Study the drawing (mm; zero at the part's minimum x, y, z) and answer. Round coordinates to 2 decimals unless told otherwise and drop trailing zeros. Loops run counter-clockwise (first coordinate to the right, second up) from the corner with the lowest first, then second, coordinate; pieces in that order, holes last. Notation, with made-up numbers: (70.5, -29) -> (115.5, -29) arc R30 ccw to (115.5, -2) -> close; hole circle Ø9 at (69, 9). An arc over 180 degrees is marked (long way). Write each question's results on one line, items separated by ' | '. Start each with the question number.
(1) The part is cut by section A-A (y = 2.5). Count the separate pieces of the cut face and the enclosed holes in it, plus the area to 3 significant figures.
(2) The part is cut by section C-C (z = 41). Determine the outline of the cut face in (x, y), plus the area to 3 significant figures.
(3) Straight lines are drawn through the part: probe 1 along Z at (x, y) = (123, 6.25); probe 2 along Z at (x, y) = (98, 2.25). For each, find the intervals that lie inside material, in ascending order.
(4) Flat-ended cylindrical pins translate along their axes: pin 1 (1.5 mm diameter, centred on y = 2.5, z = 28, fed in from +X); pin 2 (3 mm diameter, centred on y = 0.5, z = 47, fed in from +X); pin 3 (3 mm diameter, centred on y = 5.5, z = 72, fed in from +X). Find the tip coordinate at first contact, or state that the pin passes through.
(5) The part is cut by section B-B (x = 156.5). Determine the outline of the cut face in (y, z), plus the area to 3 significant figures.
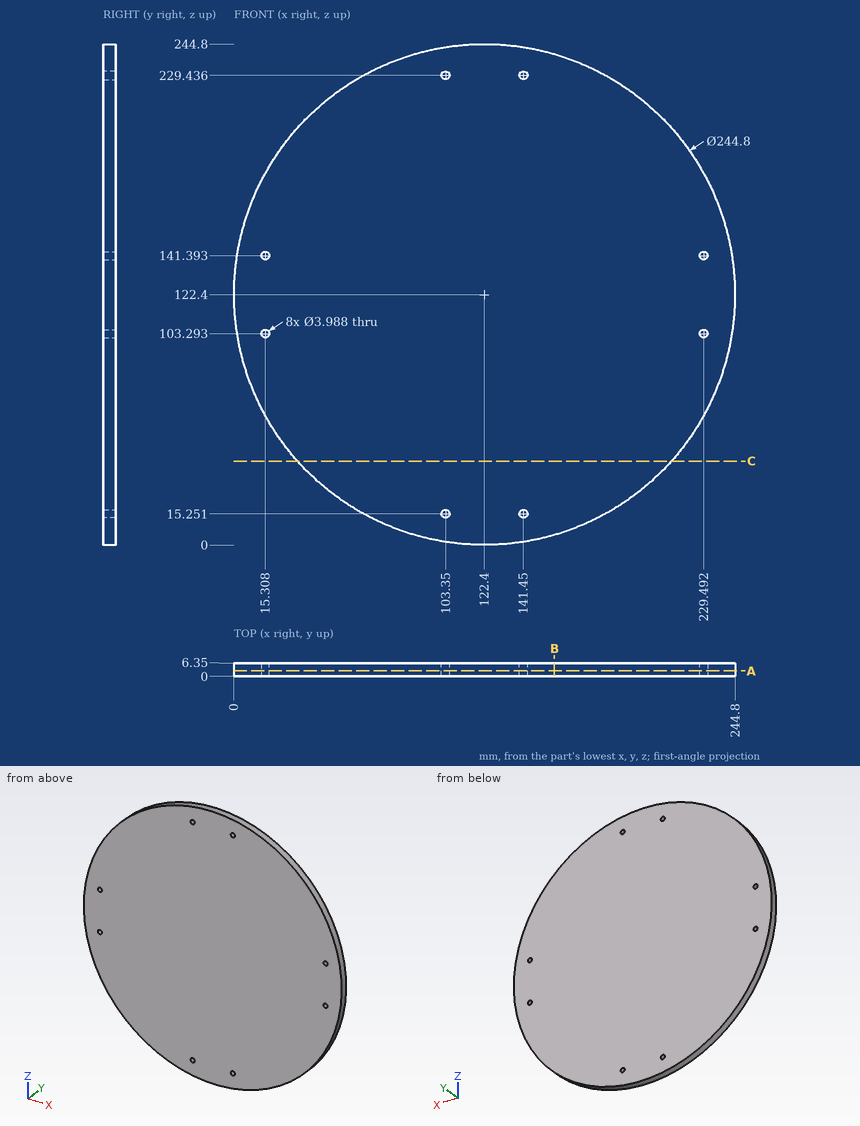
Checked values:
1) separate pieces: 1 | enclosed holes: 8 | area: 47,000 mm2
2) outline: (30.99, 0) -> (213.81, 0) -> (213.81, 6.35) -> (30.99, 6.35) -> close | area: 1,160 mm2
3) probe 1: z = 0 to 244.8 | probe 2: z = 2.46 to 242.34
4) pin 1: stops at x = 201.21 | pin 2: stops at x = 219.97 | pin 3: stops at x = 234.61
5) outline: (0, 4.85) -> (6.35, 4.85) -> (6.35, 239.95) -> (0, 239.95) -> close | area: 1,490 mm2
